from build123d import *

# Parameters (mm, degrees)
F2_R     = 10.4775
F2_R_2   = 9.2075
F3_DEPTH = 25.4
F4_DEPTH = 25.4
F5_W     = 41.00275971
F5_H     = 25.6858672947
F6_DEPTH = 127
F7_W     = 46.4864122256
F7_H     = 46.355
F8_DEPTH = 2.54


with BuildPart() as f3:
    # F2 (on line) → F3 (new body)
    with BuildSketch(Plane(origin=(0, 0, 0), x_dir=(0.9937679192, 0, 0.1114689322), z_dir=(0.1114689322, 0, -0.9937679192))):
        with Locations((41.0343617785, 0)):
            Circle(F2_R)
        with Locations((41.0343617785, 0)):
            Circle(F2_R_2, mode=Mode.SUBTRACT)
    extrude(amount=-F3_DEPTH)

    # F4 (add): a face of the model
    f4_faces = [f3.faces().sort_by_distance(p)[0] for p in [
        (30.6609305302, 0, 3.4391743995),
    ]]
    extrude(f4_faces, amount=F4_DEPTH)

    # F5 (on Front) → F6 (cut, symmetric)
    with BuildSketch(Plane.XZ):
        with Locations((39.3967321143, -12.8429336473)):
            Rectangle(F5_W, F5_H)
    extrude(amount=F6_DEPTH, both=True, mode=Mode.SUBTRACT)

    # F7 (on Top) → F8 (join)
    with BuildSketch(Plane.XY):
        with Locations((41.2916949595, 0)):
            Rectangle(F7_W, F7_H)
    extrude(amount=-F8_DEPTH)


solid = f3.part
Can you work these out from the model? Positions are in its coordinate system, mm. Round coordinates to 2 decimals unless told otherwise and drop trailing zeros. Write each loop counter-clockwise with the first axis right and the second up, starting at its lowest first coordinate (ties: lowest second). Pieces come first, ordered by that corner, then holes. Notation, with made-up numbers: M -22,49 L -6,49 A12 cw -6,62 Z; hole C 61.5,79.5 d9. An arc over 180 degrees is marked long. Use CSV: the item, a comma, the result in double quotes.
(1) Imagine slicing it at C-C (y = -4). Write out the boundary of the cut face in (x, z).
Check values:
outline,"M 18.05,-2.54 L 64.53,-2.54 L 64.53,0 L 51.04,0 L 47.57,30.9 L 46.19,30.74 L 49.64,0 L 32.95,0 L 29.71,28.89 L 28.32,28.74 L 31.55,0 L 18.05,0 Z"
(2) Imagine slicing it at A-A (y = 2.5). Write out the boundary of the cut face in (x, z).
Check values:
outline,"M 18.05,-2.54 L 64.53,-2.54 L 64.53,0 L 51.53,0 L 48.06,30.95 L 46.75,30.8 L 50.21,0 L 32.37,0 L 29.14,28.83 L 27.84,28.68 L 31.05,0 L 18.05,0 Z"
(3) Imagine slicing it at B-B (x = 24.5). Write out the boundary of the cut face in (y, z).
Check values:
outline,"M -23.18,-2.54 L 23.18,-2.54 L 23.18,0 L -23.18,0 Z"
(4) We'd pull the mould along X, two halves only. Please class faces 1 (the flat face through (41, 0, 0)), 2 (the flat face through (64.535, 0, -1)), 3 (the flat face through (18.048, 0, -1)): +X half, -X half, draft (parallel to the pull), parting line (faces both ways), or undercut.
Check values:
face 1,"undercut"
face 2,"+X half"
face 3,"-X half"
(5) I'm going to push flat-ended pins straight in: pin 1 (20.5 mm diameter, centred on x = 43, y = 0, fed in from +Z); pin 2 (3 mm diameter, centred on x = 42, y = -1, fed in from +Z); pin 3 (4 mm diameter, centred on x = 37.5, z = 5.5, fed in from -Y); pin 4 (1 mm diameter, centred on y = -4.5, z = 10, fed in from -X). Where does each tip first touch, or does it pass through?
Check values:
pin 1,"z = 30.98"
pin 2,"z = 0"
pin 3,"y = -10.41"
pin 4,"x = 30.42"
(6) I need wall thicknesses on line 1 along Z through (x, y) = (44, 16.5); line 2 along Y through (x, z) = (41.5, 14); line 3 along Y through (x, z) = (44, 27). Which ranges of each line are inside material? Lowest first, please.
Check values:
line 1,"-2.54 to 0"
line 2,"-10.33 to -9.04, 9.04 to 10.33"
line 3,"-8.79 to -7.23, 7.23 to 8.79"
(7) Imagine slicing it at D-D (y = 16). Write out the boundary of the cut face in (x, z), plus the area to 3 significant figures.
Check values:
outline,"M 18.05,-2.54 L 64.53,-2.54 L 64.53,0 L 18.05,0 Z"
area,"118 mm^2"
